The listing builds one solid part. Answer for the finished solid, in the listing's coordinates (mm). A direction names the side the tool comes from. Give positions to 0.01 mm unless a question says otherwise; leave off trailing zeros. Write each loop counter-clockwise with the first axis right and the second up, starting at its lowest first coordinate (ties: lowest second). Pieces come first, ordered by that corner, then holes. Notation, with made-up numbers: (16.5, -22) - (39.5, -22) arc R26 ccw to (39.5, -7) - close; hole circle Ø7 at (-38, -11.75). An arc over 180 degrees is marked (long way). Return JSON: item names as keys, results as strings.
Autodesk Inventor part; units mm, degrees
ref_plane "YZ Plane" through (0, 0, 0) normal (1, 0, 0) x (0, 1, 0)
ref_plane "XZ Plane" through (0, 0, 0) normal (0, 1, 0) x (-1, 0, 0)
ref_plane "XY Plane" through (0, 0, 0) normal (0, 0, 1) x (1, 0, 0)
sketch "Sketch1" plane through (0, 0, 0) normal (0, 0, 1) x (1, 0, 0)
  line L0 (-20, -85.8136) -> (-20, -78.3136)
  line L1 (-20, -78.3136) -> (-18.5, -78.3136)
  line L2 (-18.5, -78.3136) -> (-18.5, -82.5636)
  line L3 (-18.5, -82.5636) -> (-17.8462, -82.5636)
  line L4 (-17.8462, -82.5636) -> (-14, -78.7175)
  line L5 (-14, -78.7175) -> (-14, -72.9098)
  line L6 (-14, -72.9098) -> (-17.8462, -69.0636)
  line L7 (-17.8462, -69.0636) -> (-18.5, -69.0636)
  line L8 (-18.5, -69.0636) -> (-18.5, -73.3136)
  line L9 (-18.5, -73.3136) -> (-20, -73.3136)
  line L10 (-20, -73.3136) -> (-20, -65.8136)
  line L11 (-20, -65.8136) -> (-12.5, -65.8136)
  line L12 (-12.5, -65.8136) -> (-12.5, -67.3136)
  line L13 (-12.5, -67.3136) -> (-16.75, -67.3136)
  line L14 (-16.75, -67.3136) -> (-16.75, -68.0385)
  line L15 (-16.75, -68.0385) -> (-12.9748, -71.8136)
  line L16 (-12.9748, -71.8136) -> (-7.0252, -71.8136)
  line L17 (-7.0252, -71.8136) -> (-3.25, -68.0385)
  line L18 (-3.25, -68.0385) -> (-3.25, -67.3136)
  line L19 (-3.25, -67.3136) -> (-7.5, -67.3136)
  line L20 (-7.5, -67.3136) -> (-7.5, -65.8136)
  line L21 (-7.5, -65.8136) -> (0, -65.8136)
  line L22 (0, -65.8136) -> (0, -73.3136)
  line L23 (0, -73.3136) -> (-1.5, -73.3136)
  line L24 (-1.5, -73.3136) -> (-1.5, -69.0636)
  line L25 (-1.5, -69.0636) -> (-2.1538, -69.0636)
  line L26 (-2.1538, -69.0636) -> (-6, -72.9098)
  line L27 (-6, -72.9098) -> (-6, -78.7175)
  line L28 (-6, -78.7175) -> (-2.1538, -82.5636)
  line L29 (-2.1538, -82.5636) -> (-1.5, -82.5636)
  line L30 (-1.5, -82.5636) -> (-1.5, -78.3136)
  line L31 (-1.5, -78.3136) -> (0, -78.3136)
  line L32 (0, -78.3136) -> (0, -85.8136)
  line L33 (0, -85.8136) -> (-7.5, -85.8136)
  line L34 (-7.5, -85.8136) -> (-7.5, -84.3136)
  line L35 (-7.5, -84.3136) -> (-3.25, -84.3136)
  line L36 (-3.25, -84.3136) -> (-3.25, -83.5888)
  line L37 (-3.25, -83.5888) -> (-7.0252, -79.8136)
  line L38 (-7.0252, -79.8136) -> (-12.9748, -79.8136)
  line L39 (-12.9748, -79.8136) -> (-16.75, -83.5888)
  line L40 (-16.75, -83.5888) -> (-16.75, -84.3136)
  line L41 (-16.75, -84.3136) -> (-12.5, -84.3136)
  line L42 (-12.5, -84.3136) -> (-12.5, -85.8136)
  line L43 (-12.5, -85.8136) -> (-20, -85.8136)
  circle A0 centre (-10, -75.8136) radius 2.15
  line L44 (-12.4, -65.7136) -> (-7.6, -65.7136)
  line L45 (-7.6, -65.7136) -> (-7.6, -67.9136)
  line L46 (-7.6, -67.9136) -> (-12.4, -67.9136)
  line L47 (-12.4, -67.9136) -> (-12.4, -65.7136)
  line L48 (-12.4, -67.9136) -> (-13.9, -67.9136)
  line L49 (-7.6, -67.9136) -> (-6.1, -67.9136)
  arc A1 (-13.9, -67.9136) -> (-6.1, -67.9136) centre (-10, -67.0248) ccw
  line L50 (-20, -65.8136) -> (-20, -59.8136)
  line L51 (-14, -75.8136) -> (-32.3565, -75.8136)
  line L52 (-20, -75.8136) -> (-60.6, -75.8136)
  line L53 (-60.6, -75.8136) -> (-60.6, -57.5136)
  line L54 (-58.6, -55.5136) -> (-22, -55.5136)
  line L55 (-20, -57.5136) -> (-20, -75.8136)
  line L56 (-22, -55.5136) -> (-20, -57.5136)
  line L57 (-60.6, -57.5136) -> (-58.6, -55.5136)
  arc A2 (-27.6, -75.8136) -> (-53, -75.8136) centre (-40.3, -75.8136) ccw
  circle A3 centre (-55.3, -60.8136) radius 3.05
  circle A4 centre (-25.3, -60.8136) radius 3.05
  line L58 (-20, -65.7136) -> (-1, -65.7136)
  line L59 (-1, -65.7136) -> (-1, -61.7136)
  line L60 (-3, -59.7136) -> (-20, -59.7136)
  line L61 (-20, -59.7136) -> (-20, -65.7136)
  arc A5 (-1, -61.7136) -> (-3, -59.7136) centre (-3, -61.7136) ccw
  point P0 (0, 0)
  point P1 (-1, -65.8136)
  point P2 (-1, -59.8136)
  point P3 (-60.6, -55.5136)
  point P4 (-20, -55.5136)
  point P5 (-1, -59.7136)
  dimension "d3" = 4.8
  dimension "d4" = 2.2
  dimension "d6" = 0.1
  dimension "d7" = 1.5
  dimension "d8" = 1.5
  dimension "d9" = 4
  dimension "d10" = 19
  dimension "d11" = 6
  dimension "d15" = 40.6
  dimension "d16" = 20.3
  dimension "d17" = 2
  dimension "d18" = 2
  dimension "d19" = 2
  dimension "d20" = 2
  dimension "d21" = 25.4
  dimension "d22" = 6.1
  dimension "d23" = 5.3
  dimension "d24" = 5.3
  dimension "d25" = 6.1
  dimension "d26" = 5.3
  dimension "d27" = 5.3
  dimension "d32" = 0.6
  dimension "d33" = 19
  dimension "d34" = 6
  dimension "d35" = 2
extrude "Extrusion1" add sketch "Sketch1" along normal blind 9 contours L51 A2 L52 L53 L57 L54 L56 L55 L50 L10 | L50 L55 L60 A5 L59 L58 L44 | L44 L45 L46 L47 | L46 L49 A1 L48
sketch "Sketch4" plane through (0, 0, 0) normal (0, 0, -1) x (-1, 0, 0)
  line L0 (22, -55.5136) -> (58.6, -55.5136)
  line L1 (20, -57.5136) -> (22, -55.5136)
  line L2 (20, -59.7136) -> (20, -57.5136)
  line L3 (3, -59.7136) -> (20, -59.7136)
  arc A0 (3, -59.7136) -> (1, -61.7136) centre (3, -61.7136) ccw
  line L4 (1, -65.7136) -> (1, -61.7136)
  line L5 (7.6, -65.7136) -> (1, -65.7136)
  line L6 (7.6, -67.9136) -> (7.6, -65.7136)
  line L7 (6.1, -67.9136) -> (7.6, -67.9136)
  arc A1 (6.1, -67.9136) -> (13.9, -67.9136) centre (10, -67.0248) ccw
  line L8 (12.4, -67.9136) -> (13.9, -67.9136)
  line L9 (12.4, -65.7136) -> (12.4, -67.9136)
  line L10 (20, -65.7136) -> (12.4, -65.7136)
  line L11 (20, -75.8136) -> (20, -65.7136)
  line L12 (27.6, -75.8136) -> (20, -75.8136)
  arc A2 (53, -75.8136) -> (27.6, -75.8136) centre (40.3, -75.8136) ccw
  line L13 (60.6, -75.8136) -> (53, -75.8136)
  line L14 (60.6, -57.5136) -> (60.6, -75.8136)
  line L15 (58.6, -55.5136) -> (60.6, -57.5136)
  circle A3 centre (25.3, -60.8136) radius 3.05
  circle A4 centre (55.3, -60.8136) radius 3.05
  line L16 (20, -59.7136) -> (20, -57.5136)
  line L17 (20, -75.8136) -> (20, -65.7136)
  line L18 (20, -59.7136) -> (20, -65.7136)
  point P0 (0, 0)
extrude "Extrusion3" add sketch "Sketch4" along normal blind 9 contours L18 L10 L9 L8 A1 L7 L6 L5 L4 A0 L3
sketch "Sketch5" plane through (-20, -59.7136, 9) normal (0, 1, 0) x (1, 0, 0)
  line L0 (6.1, 18) -> (6.1, 0)
  line L1 (13.9, 18) -> (13.9, 0)
  circle A0 centre (10, 4) radius 1.95
  circle A1 centre (10, 14) radius 1.95
  line L2 (0, 18) -> (17, 18)
  line L3 (17, 0) -> (0, 0)
  point P0 (20, 9)
  dimension "d38" = 3.9
  dimension "d39" = 3.9
  dimension "d40" = 3.9
  dimension "d41" = 3.9
  dimension "d42" = 4
  dimension "d43" = 4
hole "Hole1" at (-10, -59.7136, 5) at (-10, -59.7136, -5) direction (0, -1, 0) diameter 3.9 end through all counterbore diameter 7.4 counterbore depth 1
mirror "Mirror1" about plane through (-60.6, -75.8136, 0) normal (0, -1, 0) of "Extrusion1", "Extrusion3", "Hole1"
properties part number "Rain_LensHolder"
Item 1: The mould has two halves that part along X. Classify faces 4 (the face through (-6.88, -91.41, -3.01)), 5 (the face through (-7, -83.714, 0)), 6 (the face through (-20, -63, -4)), 7 (the face through (-12.4, -85, 0)): +X half, -X half, draft (parallel to the pull), parting line (faces both ways), or undercut.
Answer below:
{"face 4": "undercut", "face 5": "draft", "face 6": "-X half", "face 7": "undercut"}
Item 2: Flat-ended cylindrical pins translate along their axes: P1, Ø8.5, axis at x = -10, z = 5, coming from the -Y side; P2, Ø1.5, axis at x = -20, z = 4.5, coming from the -Y side; P3, Ø8, axis at x = -9, z = 6.5, coming from the +Y side. Find the tip coordinate at first contact, or state that the pin passes through.
Answer below:
{"P1": "stops at y = -91.91", "P2": "stops at y = -94.86", "P3": "stops at y = -59.71"}
Item 3: A cutting plane is placed at B-B on x = -40.3. Determine the outline of the cut face in (y, z).
Answer below:
{"outline": "(-96.11, 0) - (-88.51, 0) - (-88.51, 9) - (-96.11, 9) - close; (-63.11, 0) - (-55.51, 0) - (-55.51, 9) - (-63.11, 9) - close"}
Item 4: Consider L1, parallel to Y at x = -25.3, z = 5.25; L2, parallel to Z at x = -10, y = -64; L3, parallel to Y at x = -10, z = 1. Determine where each line is inside the solid, lowest interval first.
Answer below:
{"L1": "y = -96.11 to -93.86, -87.76 to -63.86, -57.76 to -55.51", "L2": "z = -9 to -6.95, -3.05 to 3.05, 6.95 to 9", "L3": "y = -91.91 to -80.6, -71.02 to -59.71"}
Item 5: For faces 1 (the face through (-20, -59, 4)), 2 (the face through (-20, -76, 4)), 3 (the face through (-20, -93, 4)), determine the directions among +Z, -Z, +X, -X, +Y, -Y from which every point of the face is accessible in a straight line to the end or side of a thin tool.
Answer below:
{"face 1": "+Z, -Z, +X, +Y", "face 2": "+Z, -Z", "face 3": "+Z, -Z, +X, -Y"}
Item 6: A cutting plane is placed at C-C on x = -55.3. Determine the outline of the cut face in (y, z).
Answer below:
{"outline": "(-96.11, 0) - (-93.86, 0) - (-93.86, 9) - (-96.11, 9) - close; (-87.76, 0) - (-63.86, 0) - (-63.86, 9) - (-87.76, 9) - close; (-57.76, 0) - (-55.51, 0) - (-55.51, 9) - (-57.76, 9) - close"}
Item 7: A cutting plane is placed at D-D on y = -82. Determine the outline of the cut face in (x, z).
Answer below:
{"outline": "(-60.6, 0) - (-51.39, 0) - (-51.39, 9) - (-60.6, 9) - close; (-29.21, 0) - (-20, 0) - (-20, 9) - (-29.21, 9) - close; (-13.04, -9) - (-6.96, -9) - (-6.96, 9) - (-13.04, 9) - close; hole circle Ø3.9 at (-10, -5); hole circle Ø3.9 at (-10, 5)"}
Item 8: A cutting plane is placed at A-A on y = -65. Determine the outline of the cut face in (x, z), then the cut area to 3 significant figures.
Answer below:
{"outline": "(-60.6, 0) - (-46.96, 0) - (-46.96, 9) - (-60.6, 9) - close; (-33.64, 0) - (-20, 0) - (-20, -9) - (-1, -9) - (-1, 9) - (-33.64, 9) - close; hole circle Ø3.9 at (-10, -5); hole circle Ø3.9 at (-10, 5)", "area": "564 mm²"}
